Source: CAD feature listing. Evaluate the final solid. Frame: model axes, mm. Face numbers are marked on the shaded views. A direction names the side the tool comes from. Coordinates: 2 decimals unless noted, no trailing zeros. Loops run counter-clockwise (first coordinate to the right, second up) from the corner with the lowest first, then second, coordinate; pieces in that order, holes last.
Item 1: Section query B-B, the plane y = 8. Return the cut outline in (x, z).
Item 2: Pin query (flat end, axial travel): pin 1 Ø6 at (x, y) = (1, 7.5) entering from +Z; pin 2 Ø3 at (x, z) = (-3, 60) entering from +Y; pin 3 Ø4 at (x, y) = (15.5, -15.5) entering from +Z. Return the tip coordinate at first contact, or that it passes through.
Item 3: Section query C-C, the plane z = 41. Return the cut outline in (x, y), then the cut area to 3 significant figures.
Item 4: Line query: probe 1 along X at (y, z) = (-15.5, 36); probe 2 along Z at (x, y) = (10, -3.5). Output: solid intervals per line, ascending.
Item 5: Section query D-D, the plane z = 68. Return the cut outline in (x, y), then the cut area to 3 significant figures.
Item 6: Section query A-A, the plane z = 9.5. Return the cut outline in (x, y), then the cut area to 3 significant figures.
Item 7: Reachability of the marked faces 1 and 2 from +Z, -Z, +X, -X, +Y, -Y: full face, straight path, thin tool, end or side. Return the list, or none.
```python
from build123d import *

# Parameters (mm, degrees)
F0_W      = 42
F0_H      = 42
F1_DEPTH  = 39
F2_R      = 16
F3_DEPTH  = 22.1
F4_R      = 10
F5_DEPTH  = 3
F6_R      = 3
F7_DEPTH  = 16.3
F8_SIZE   = 5.5
F10_D     = 3.3
F10_DEPTH = 7
F10_TIP   = 0.9914200214
F12_D     = 3.4
F12_DEPTH = 7
F12_TIP   = 1.0214630523


with BuildPart() as f1:
    # F0 (on Top) → F1 (new body)
    with BuildSketch(Plane.XY):
        Rectangle(F0_W, F0_H)
    extrude(amount=F1_DEPTH)

    # F2 (on face) → F3 (join)
    with BuildSketch(Plane.XY.offset(39)):
        Circle(F2_R)
    extrude(amount=F3_DEPTH)

    # F4 (on face) → F5 (join)
    with BuildSketch(Plane.XY.offset(61.1)):
        Circle(F4_R)
    extrude(amount=F5_DEPTH)

    # F6 (on face) → F7 (join)
    with BuildSketch(Plane.XY.offset(64.1)):
        Circle(F6_R)
    extrude(amount=F7_DEPTH)

    # F8
    f8_edges = [f1.edges().sort_by_distance(p)[0] for p in [
        (-21, 21, 19.5),
        (21, 21, 19.5),
        (21, -21, 19.5),
        (-21, -21, 19.5),
    ]]
    chamfer(f8_edges, length=F8_SIZE)

    # F10
    with Locations(Plane.XY.offset(39)):
        with Locations((-15.5, 15.5), (15.5, 15.5), (15.5, -15.5), (-15.5, -15.5)):
            Hole(F10_D / 2, depth=F10_DEPTH)
            with Locations((0, 0, -(F10_DEPTH + F10_TIP / 2))):  # 118° drill point
                Cone(0, F10_D / 2, F10_TIP, mode=Mode.SUBTRACT)

    # F12
    with Locations(Plane.XY.offset(61.1)):
        with Locations((0, 13), (-13, 0), (0, -13), (13, 0)):
            Hole(F12_D / 2, depth=F12_DEPTH)
            with Locations((0, 0, -(F12_DEPTH + F12_TIP / 2))):  # 118° drill point
                Cone(0, F12_D / 2, F12_TIP, mode=Mode.SUBTRACT)


solid = f1.part
```
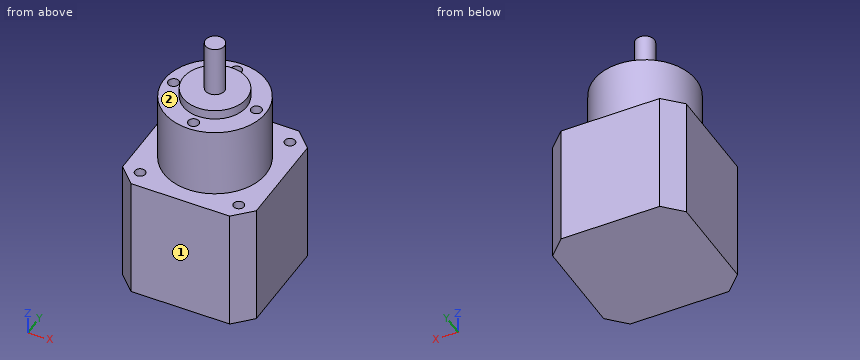
Verdict:
1. outline: (-21, 0) - (21, 0) - (21, 39) - (13.86, 39) - (13.86, 61.1) - (6, 61.1) - (6, 64.1) - (-6, 64.1) - (-6, 61.1) - (-13.86, 61.1) - (-13.86, 39) - (-21, 39) - close
2. pin 1: stops at z = 64.1
2. pin 2: stops at y = 15.93
2. pin 3: stops at z = 39
3. outline: circle Ø32 at (0, 0)
3. area: 804 mm2
4. probe 1: x = -21 to -17.15, -13.85 to 13.85, 17.15 to 21
4. probe 2: z = 0 to 61.1
5. outline: circle Ø6 at (0, 0)
5. area: 28.3 mm2
6. outline: (-21, -15.5) - (-15.5, -21) - (15.5, -21) - (21, -15.5) - (21, 15.5) - (15.5, 21) - (-15.5, 21) - (-21, 15.5) - close
6. area: 1,700 mm2
7. face 1: +Z, -Z, +X, -X, -Y
7. face 2: +Z
